Autodesk Inventor part; units mm, degrees
ref_plane "YZ Plane" through (0, 0, 0) normal (1, 0, 0) x (0, 1, 0)
ref_plane "XZ Plane" through (0, 0, 0) normal (0, 1, 0) x (-1, 0, 0)
ref_plane "XY Plane" through (0, 0, 0) normal (0, 0, 1) x (1, 0, 0)
sketch "Sketch1" plane through (0, 0, 0) normal (0, 0, 1) x (1, 0, 0)
  line L0 (-80.9183, 81.3988) -> (69.0817, 81.3988)
  line L1 (69.0817, 81.3988) -> (69.0817, -68.6012)
  line L2 (69.0817, -68.6012) -> (-80.9183, -68.6012)
  line L3 (-80.9183, -68.6012) -> (-80.9183, 81.3988)
  line L4 (-80.9183, 81.3988) -> (69.0817, -68.6012) construction
  line L5 (69.0817, 81.3988) -> (-80.9183, -68.6012) construction
  point P0 (0, 0)
  point P1 (-5.9183, 6.3988)
  dimension "d0" = 150
  dimension "d1" = 150
extrude "Extrusion1" add sketch "Sketch1" along normal blind 100
sketch "Sketch2" plane through (0, 0, 100) normal (0, 0, 1) x (1, 0, 0)
  circle A0 centre (-4.4387, 8.6963) radius 40
  point P0 (0, 0)
  dimension "d4" = 80
extrude "Extrusion2" add sketch "Sketch2" along normal blind 120
sketch "Sketch3" plane through (-4.4387, 8.6963, 220) normal (0, 0, 1) x (1, 0, 0)
  line L0 (-210, 40) -> (210, 40)
  line L1 (210, 40) -> (210, -40)
  line L2 (210, -40) -> (-210, -40)
  line L3 (-210, -40) -> (-210, 40)
  circle A0 centre (0, 0) radius 40
  line L4 (-210, 40) -> (210, -40) construction
  line L5 (210, 40) -> (-210, -40) construction
  point P0 (4.4387, -8.6963)
  dimension "d7" = 420
  dimension "d8" = 80
extrude "Extrusion3" add sketch "Sketch3" along normal blind 80
sketch "Sketch4" plane through (-4.4387, 8.6963, 300) normal (0, 0, 1) x (1, 0, 0)
  line L0 (210, 40) -> (-210, 40)
  line L1 (-210, -40) -> (210, -40)
  line L2 (-210, 40) -> (-130, 40)
  line L3 (-130, 40) -> (-130, -40)
  line L4 (-130, -40) -> (-210, -40)
  line L5 (-210, -40) -> (-210, 40)
  line L6 (210, -40) -> (210, 40)
  line L7 (210, 40) -> (130, 40)
  line L8 (130, 40) -> (130, -40)
  line L9 (130, -40) -> (210, -40)
  line L10 (210, -40) -> (210, 40)
  point P0 (4.4387, -8.6963)
  point P1 (130, 40)
  dimension "d11" = 80
  dimension "d12" = 80
extrude "Extrusion4" add sketch "Sketch4" along normal blind 90 contours L6 L1 L8 L0 | L3 L1 L5 L0
sketch "Sketch5" plane through (69.0817, -68.6012, 0) normal (1, 0, 0) x (0, 0, -1)
  circle A0 centre (-49.808, 76.4656) radius 25
  point P0 (0, 68.6012)
  dimension "d15" = 50
extrude "Extrusion5" cut sketch "Sketch5" against normal blind 500
properties part number "HOLDER"
Part model, mm, in its own coordinate system. A direction names the side the tool comes from. Round coordinates to 2 decimals unless told otherwise and drop trailing zeros. Write each loop counter-clockwise with the first axis right and the second up, starting at its lowest first coordinate (ties: lowest second). Pieces come first, ordered by that corner, then holes.
Item 1: Cut at B-B, the plane y = 20. Give the cut face in (x, z).
Results:
outline: (-214.44, 220) - (-42.81, 220) - (-42.81, 100) - (-80.92, 100) - (-80.92, 71.66) - (69.08, 71.66) - (69.08, 100) - (33.93, 100) - (33.93, 220) - (205.56, 220) - (205.56, 390) - (125.56, 390) - (125.56, 300) - (-134.44, 300) - (-134.44, 390) - (-214.44, 390) - close; (-80.92, 0) - (69.08, 0) - (69.08, 27.95) - (-80.92, 27.95) - close
Item 2: Drop flat-ended pins along their axis: pin 1 Ø12 at (y, z) = (14.5, 188.5) entering from +X; pin 2 Ø8 at (x, z) = (-0.5, 151.5) entering from -Y; pin 3 Ø8 at (y, z) = (44, 199.5) entering from +X. Give the stop position or say it passes through.
Results:
pin 1: stops at x = 35.56
pin 2: stops at y = -31.3
pin 3: stops at x = 20.46
Item 3: Two-plate mould, pull along Z, no slides. Class faces 1 (the cylindrical face through (-4.868, 8.964, 74.784)), 2 (the flat face through (165, 9, 390)), 3 (the flat face through (69.082, -9, 27)): +Z half, -Z half, draft (parallel to the pull), parting line (faces both ways), or undercut.
Results:
face 1: undercut
face 2: +Z half
face 3: draft
Item 4: Cut at D-D, the plane z = 229.5. Give the cut face in (x, y), plus the area to 3 significant figures.
Results:
outline: (-214.44, -31.3) - (205.56, -31.3) - (205.56, 48.7) - (-214.44, 48.7) - close
area: 33,600 mm2
Item 5: Which spindle directions (+Z, -Z, +X, -X, +Y, -Y) get a long thin tool onto all of the face, cutting with end or side? Do faces 4 (the flat face through (-7, 48.696, 285)), 5 (the cylindrical face through (33.714, -3.319, 159.16)), 6 (the flat face through (-1, -31.304, 285)). Say none if no direction does.
Results:
face 4: +Z, +X, -X, +Y
face 5: none
face 6: +Z, +X, -X, -Y
Item 6: Probe L1, parallel to X at y = -13, z = 312.5; L2, parallel to Z at x = 128, y = -10.5; L3, parallel to Y at x = 173, z = 352. List the from-to ranges inside material, lowest first.
Results:
L1: x = -214.44 to -134.44, 125.56 to 205.56
L2: z = 220 to 390
L3: y = -31.3 to 48.7
Item 7: Cut at A-A, the plane z = 322.5. Give the cut face in (x, y), plus the area to 3 significant figures.
Results:
outline: (-214.44, -31.3) - (-134.44, -31.3) - (-134.44, 48.7) - (-214.44, 48.7) - close; (125.56, -31.3) - (205.56, -31.3) - (205.56, 48.7) - (125.56, 48.7) - close
area: 12,800 mm2
Item 8: Cut at C-C, the plane x = 24. Give the cut face in (y, z), plus the area to 3 significant figures.
Results:
outline: (-68.6, 0) - (81.4, 0) - (81.4, 100) - (36.83, 100) - (36.83, 220) - (48.7, 220) - (48.7, 300) - (-31.3, 300) - (-31.3, 220) - (-19.43, 220) - (-19.43, 100) - (-68.6, 100) - close; hole circle Ø50 at (7.86, 49.81)
area: 26,200 mm2
